Job drawing, mm, ordinate dimensions from the low corner. One solid piece. Coordinates: 2 decimals unless noted, no trailing zeros. Loops run counter-clockwise (first coordinate to the right, second up) from the corner with the lowest first, then second, coordinate; pieces in that order, holes last. Notation, with made-up numbers: (75, -20.5) - (124, -20.5) arc R8 cw to (124, -7.5) - close; hole circle Ø2 at (45, 66.25). An arc over 180 degrees is marked (long way). Use a Markdown table: item, result. Add a question column.
1. Pull direction Y, two halves, no side cores. Call the marked faces 1, 2 and 3: pulls with the +Y half, pulls with the -Y half, needs draft (parallel to the pull), parting line crosses it, or undercut.
2. Band-saw the part on A-A, the plane x = 11.5. Give the cut face in (y, z) (1 decimal), plus the area to 3 significant figures.
3. Band-saw the part on B-B, the plane y = 10. Give the cut face in (x, z) (1 decimal).
4. Band-saw the part on D-D, the plane z = 5.75. Give the cut face in (x, y) (1 decimal).
5. Band-saw the part on C-C, the plane x = 5.75. Give the cut face in (y, z), plus the area to 3 significant figures.
6. Drop flat-ended pins along their axis: pin 1 (6.5 mm diameter, centred on x = 12, y = 9.5, fed in from +Z); pin 2 (10 mm diameter, centred on y = 2, z = 9, fed in from -X); pin 3 (2 mm diameter, centred on x = 3, z = 6, fed in from +Y) (1 decimal). Give the stop position or say it passes through.
7. Wall check: probe 1 along Z at (x, y) = (1.5, 14); probe 2 along Y at (x, z) = (7, 16.25); probe 3 along Y at (x, z) = (6.5, 6.75) (1 decimal). Give the ranges that are in metal, low to high. Write a range as [from, to].
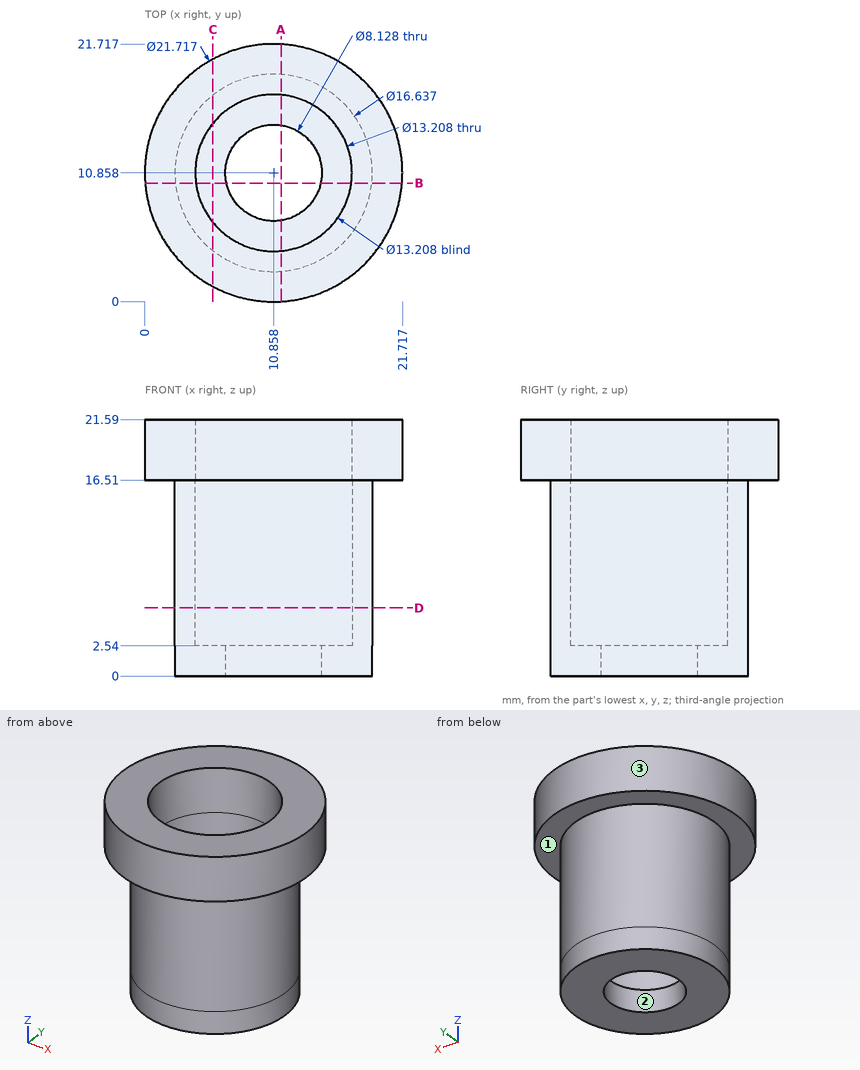
Geometry check:
| question | item | result |
|---|---|---|
| 1 | face 1 | needs draft |
| 1 | face 2 | undercut |
| 1 | face 3 | parting line crosses it |
| 2 | outline | (0, 16.5) - (2.6, 16.5) - (2.6, 0) - (6.8, 0) - (6.8, 2.5) - (4.3, 2.5) - (4.3, 21.6) - (0, 21.6) - close; (14.9, 0) - (19.2, 0) - (19.2, 16.5) - (21.7, 16.5) - (21.7, 21.6) - (17.4, 21.6) - (17.4, 2.5) - (14.9, 2.5) - close |
| 2 | area | 113 mm^2 |
| 3 | outline | (0, 16.5) - (2.6, 16.5) - (2.6, 0) - (6.9, 0) - (6.9, 2.5) - (4.3, 2.5) - (4.3, 21.6) - (0, 21.6) - close; (14.8, 0) - (19.1, 0) - (19.1, 16.5) - (21.7, 16.5) - (21.7, 21.6) - (17.4, 21.6) - (17.4, 2.5) - (14.8, 2.5) - close |
| 4 | outline | circle Ø16.6 at (10.9, 10.9); hole circle Ø13.2 at (10.9, 10.9) |
| 5 | outline | (1.28, 16.51) - (4.29, 16.51) - (4.29, 0) - (17.42, 0) - (17.42, 16.51) - (20.44, 16.51) - (20.44, 21.59) - (15.04, 21.59) - (15.04, 2.54) - (6.67, 2.54) - (6.67, 21.59) - (1.28, 21.59) - close |
| 5 | area | 155 mm^2 |
| 6 | pin 1 | stops at z = 2.54 |
| 6 | pin 2 | stops at x = 3.49 |
| 6 | pin 3 | stops at y = 15.6 |
| 7 | probe 1 | z = [16.51, 21.59] |
| 7 | probe 2 | y = [3.49, 5.5], [16.22, 18.23] |
| 7 | probe 3 | y = [3.8, 5.9], [15.8, 17.9] |
